```python
from build123d import *

# Parameters (mm, degrees)
SKETCH1_R                = 31.543
SKETCH1_R_2              = 26.543
BOSS_EXTRUDE1_DEPTH      = 10
SKETCH2_W                = 100
SKETCH2_H                = 82
BOSS_EXTRUDE2_DEPTH      = 5
M4_CLEARANCE_HOLE2_D     = 4.5
M4_CLEARANCE_HOLE2_DEPTH = 5
SKETCH8_R                = 31.543
SKETCH8_R_2              = 26.543
BOSS_EXTRUDE3_DEPTH      = 65


with BuildPart() as part:
    # Sketch1 → Boss-Extrude1 (new body)
    with BuildSketch(Plane.XY):
        Circle(SKETCH1_R)
        Circle(SKETCH1_R_2, mode=Mode.SUBTRACT)
    extrude(amount=-BOSS_EXTRUDE1_DEPTH)

    # Sketch2 → Boss-Extrude2 (add)
    with BuildSketch(Plane.XY):
        Rectangle(SKETCH2_W, SKETCH2_H)
    extrude(amount=BOSS_EXTRUDE2_DEPTH)

    # M4 Clearance Hole2
    with Locations(Plane(origin=(0, 0, 0), x_dir=(-1, 0, 0), z_dir=(0, 0, -1))):
        with Locations((-40, 31.543), (40, 31.543), (40, -31.543), (-40, -31.543)):
            Hole(M4_CLEARANCE_HOLE2_D / 2, depth=M4_CLEARANCE_HOLE2_DEPTH)

    # Sketch8 → Boss-Extrude3 (add)
    with BuildSketch(Plane.XY.offset(5)):
        Circle(SKETCH8_R)
        Circle(SKETCH8_R_2, mode=Mode.SUBTRACT)
    extrude(amount=BOSS_EXTRUDE3_DEPTH)


solid = part.part
```
Verification items for the finished model (mm, model axes). A direction names the side the tool comes from. Round coordinates to 2 decimals unless told otherwise and drop trailing zeros. Write each loop counter-clockwise with the first axis right and the second up, starting at its lowest first coordinate (ties: lowest second). Pieces come first, ordered by that corner, then holes.
1. Gauge pin test, flat ends, axial feed: P1, Ø3, axis at x = 22, y = 30, coming from the +Z side; P2, Ø2.5, axis at x = -40, y = -31.543, coming from the +Z side; P3, Ø8, axis at y = -13, z = 35.5, coming from the -X side; P4, Ø1, axis at y = 6, z = 9.5, coming from the -X side. Record the tip position at first contact, or that the pin passes through.
2. Section check B-B on x = 40. Enter the section's corners in (y, z).
3. Section check D-D on y = 13. Enter the section's corners in (x, z).
4. Scan lines: L1, parallel to Y at x = -40, z = 1.25; L2, parallel to Z at x = 32.5, y = 6.5; L3, parallel to X at y = 4, z = 24.5. Record each from-to range of solid material in increasing order.
5. Section check C-C on z = 61.5. Enter the section's corners in (x, y), plus the area to 3 significant figures.
6. Section check A-A on x = 0. Enter the section's corners in (y, z), plus the area to 3 significant figures.
7. Draft check along X on faces 4 (the cylindrical face through (-6.8, -30.8, -4.9)), 5 (the cylindrical face through (12.248, -23.548, -4.93)), 6 (the flat face through (-50, -1, 2)), 7 (the flat face through (-34, 1, 0)). Enter one of: +X half, -X half, draft (parallel to the pull), parting line (faces both ways), or undercut.
8. Access from +Z, -Z, +X, -X, +Y, -Y to the whole of each face (thin tool, end or side, straight path). Record for faces 1 (the flat face through (0, 0, 0)), 2 (the cylindrical face through (39.71, -29.31, 2.54)), 3 (the cylindrical face through (12.248, -23.548, 37.045)).
Answer:
1. P1: stops at z = 5
1. P2: passes through
1. P3: stops at x = -30.23
1. P4: stops at x = -31.06
2. outline: (-41, 0) - (-33.79, 0) - (-33.79, 5) - (-41, 5) - close; (-29.29, 0) - (29.29, 0) - (29.29, 5) - (-29.29, 5) - close; (33.79, 0) - (41, 0) - (41, 5) - (33.79, 5) - close
3. outline: (-50, 0) - (-28.74, 0) - (-28.74, -10) - (-23.14, -10) - (-23.14, 0) - (23.14, 0) - (23.14, -10) - (28.74, -10) - (28.74, 0) - (50, 0) - (50, 5) - (28.74, 5) - (28.74, 70) - (23.14, 70) - (23.14, 5) - (-23.14, 5) - (-23.14, 70) - (-28.74, 70) - (-28.74, 5) - (-50, 5) - close
4. L1: y = -41 to -33.79, -29.29 to 29.29, 33.79 to 41
4. L2: z = 0 to 5
4. L3: x = -31.29 to -26.24, 26.24 to 31.29
5. outline: circle Ø63.09 at (0, 0); hole circle Ø53.09 at (0, 0)
5. area: 912 mm2
6. outline: (-41, 0) - (-31.54, 0) - (-31.54, -10) - (-26.54, -10) - (-26.54, 0) - (26.54, 0) - (26.54, -10) - (31.54, -10) - (31.54, 0) - (41, 0) - (41, 5) - (31.54, 5) - (31.54, 70) - (26.54, 70) - (26.54, 5) - (-26.54, 5) - (-26.54, 70) - (-31.54, 70) - (-31.54, 5) - (-41, 5) - close
6. area: 1,160 mm2
7. face 4: parting line
7. face 5: undercut
7. face 6: -X half
7. face 7: draft
8. face 1: -Z
8. face 2: +Z, -Z
8. face 3: +Z
